Work out the finished part from the listing and answer in its coordinate system (mm). A direction names the side the tool comes from. Coordinates: 2 decimals unless noted, no trailing zeros. Loops run counter-clockwise (first coordinate to the right, second up) from the corner with the lowest first, then second, coordinate; pieces in that order, holes last. Notation, with made-up numbers: (26.25, -30) -> (50.25, -30) arc R14 cw to (50.25, -3) -> close; hole circle Ø6 at (45, -17.75). An arc over 180 degrees is marked (long way). Use a Markdown table: item, result.
from build123d import *

# Parameters (mm, degrees)
SKETCH1_R            = 5.5
SKETCH1_R_2          = 1.5
BOSS_EXTRUDE1_DEPTH  = 15
SKETCH3_W            = 9.999397818
SKETCH3_H            = 22.225224056
CUT_EXTRUDE1_DEPTH   = 5
FILLET1_R            = 1
FILLET1_OF_MIRROR1_R = 1
SKETCH4_R            = 7.5
BOSS_EXTRUDE2_DEPTH  = 3
SKETCH5_W            = 22
SKETCH5_H            = 7
CUT_EXTRUDE2_DEPTH   = 30.75172255
SKETCH6_R            = 4.5
CUT_EXTRUDE3_DEPTH   = 26.34097462
SKETCH7_R            = 4.5
CUT_EXTRUDE8_DEPTH   = 3
FILLET3_R            = 0.5
FILLET2_R            = 0.5


with BuildPart() as part:
    # Sketch1 → Boss-Extrude1 (new body)
    with BuildSketch(Plane.XY):
        with BuildLine():
            Line((-14.334802826, 9), (14.334802826, 9))
            ThreePointArc((14.334802826, 9), (17.163229951, 7.828427125), (18.334802826, 5))
            Line((18.334802826, 5), (18.334802826, -5))
            ThreePointArc((18.334802826, -5), (17.163229951, -7.828427125), (14.334802826, -9))
            Line((14.334802826, -9), (-14.334802826, -9))
            ThreePointArc((-14.334802826, -9), (-17.163229951, -7.828427125), (-18.334802826, -5))
            Line((-18.334802826, -5), (-18.334802826, 5))
            ThreePointArc((-18.334802826, 5), (-17.163229951, 7.828427125), (-14.334802826, 9))
        make_face()
        Circle(SKETCH1_R, mode=Mode.SUBTRACT)
        with Locations((-14.334802826, 0)):
            Circle(SKETCH1_R_2, mode=Mode.SUBTRACT)
        with Locations(Location((14.334802826, 0, 0), (0, 0, 180))):
            Circle(SKETCH1_R_2, mode=Mode.SUBTRACT)
    extrude(amount=BOSS_EXTRUDE1_DEPTH)

    # Sketch3 → Cut-Extrude1 (cut)
    with BuildSketch(Plane.XY.offset(15)):
        with Locations((-14.334501735, -0.429661625)):
            Rectangle(SKETCH3_W, SKETCH3_H)
    cut_extrude1 = extrude(amount=-CUT_EXTRUDE1_DEPTH, mode=Mode.SUBTRACT)

    # Fillet1
    fillet1_edges = [part.edges().sort_by_distance(p)[0] for p in [
        (-9.334802826, -9, 12.5),
        (-9.334802826, 0, 10),
        (-9.334802826, 9, 12.5),
        (-17.163229951, 7.828427125, 10),
        (-11.834802826, 9, 10),
        (-11.834802826, -9, 10),
        (-17.163229951, -7.828427125, 10),
        (-18.334802826, 0, 10),
        (-9.334802826, 0, 15),
    ]]
    fillet(fillet1_edges, radius=FILLET1_R)

    # Mirror1: Cut-Extrude1 across plane
    add(cut_extrude1.mirror(Plane(origin=(0, 0, 0), x_dir=(0, 0, 1), z_dir=(1, 0, 0))), mode=Mode.SUBTRACT)

    # Fillet1 of Mirror1
    fillet1_of_mirror1_edges = [part.edges().sort_by_distance(p)[0] for p in [
        (9.334802826, -9, 12.5),
        (9.334802826, 0, 10),
        (9.334802826, 9, 12.5),
        (17.163229951, 7.828427125, 10),
        (11.834802826, 9, 10),
        (11.834802826, -9, 10),
        (17.163229951, -7.828427125, 10),
        (18.334802826, 0, 10),
        (9.334802826, 0, 15),
    ]]
    fillet(fillet1_of_mirror1_edges, radius=FILLET1_OF_MIRROR1_R)

    # Sketch4 → Boss-Extrude2 (add)
    with BuildSketch(Plane.XY.offset(15)):
        Circle(SKETCH4_R)
    extrude(amount=-BOSS_EXTRUDE2_DEPTH)

    # Sketch5 → Cut-Extrude2 (cut, through all)
    with BuildSketch(Plane(origin=(0, 9, 0), x_dir=(1, 0, 0), z_dir=(0, 1, 0))):
        Rectangle(SKETCH5_W, SKETCH5_H)
    extrude(amount=-CUT_EXTRUDE2_DEPTH, mode=Mode.SUBTRACT)

    # Sketch6 → Cut-Extrude3 (cut, through all)
    with BuildSketch(Plane.XY.offset(15)):
        Circle(SKETCH6_R)
    extrude(amount=-CUT_EXTRUDE3_DEPTH, mode=Mode.SUBTRACT)

    # Sketch7 → Cut-Extrude8 (cut)
    with BuildSketch(Plane.XY.offset(10)):
        with Locations((-14.530374954, 0)):
            Circle(SKETCH7_R)
        with Locations((14.530374954, 0)):
            Circle(SKETCH7_R)
    extrude(amount=-CUT_EXTRUDE8_DEPTH, mode=Mode.SUBTRACT)

    # Fillet3
    fillet3_edges = [part.edges().sort_by_distance(p)[0] for p in [
        (11, -9, 1.75),
        (0, -9, 3.5),
        (11, 0, 3.5),
        (-11, -9, 1.75),
        (-11, 0, 3.5),
        (-11, 9, 1.75),
        (0, 9, 3.5),
        (11, 9, 1.75),
    ]]
    fillet(fillet3_edges, radius=FILLET3_R)

    # Fillet2
    fillet2_edges = [part.edges().sort_by_distance(p)[0] for p in [
        (-5.5, 0, 12),
    ]]
    fillet(fillet2_edges, radius=FILLET2_R)


solid = part.part
Q1. Section C-C on z = 8.5 is taken. Determine the outline of the cut face in (x, y), and give its area (3 significant figures).
Solved:
| item | result |
|---|---|
| outline | (-18.33, -5) arc R4 ccw to (-14.33, -9) -> (14.33, -9) arc R4 ccw to (18.33, -5) -> (18.33, -2.4) arc R4.5 cw (long way) to (18.33, 2.4) -> (18.33, 5) arc R4 ccw to (14.33, 9) -> (-14.33, 9) arc R4 ccw to (-18.33, 5) -> (-18.33, 2.4) arc R4.5 cw (long way) to (-18.33, -2.4) -> close; hole circle Ø11 at (0, 0) |
| area | 429 mm² |
Q2. Consider line 1 (X direction, y = 0, z = 8); line 2 (Z direction, x = -5, y = 3.5); line 3 (Z direction, x = -16, y = -5.5). Determine where each line is inside the solid, lowest interval first. Write a range as [from, to].
Solved:
| item | result |
|---|---|
| line 1 | [-10.03, -5.5], [5.5, 10.03] |
| line 2 | [3.5, 15] |
| line 3 | [0, 10] |
Q3. Section A-A on x = 0 is taken. Determine the outline of the cut face in (y, z), and give its area (3 significant figures).
Solved:
| item | result |
|---|---|
| outline | (-9, 4) arc R0.5 ccw to (-8.5, 3.5) -> (-5.5, 3.5) -> (-5.5, 11.5) arc R0.5 cw to (-5, 12) -> (-4.5, 12) -> (-4.5, 15) -> (-9, 15) -> close; (4.5, 12) -> (5, 12) arc R0.5 cw to (5.5, 11.5) -> (5.5, 3.5) -> (8.5, 3.5) arc R0.5 ccw to (9, 4) -> (9, 15) -> (4.5, 15) -> close |
| area | 86.5 mm² |
Q4. Section B-B on z = 4.75 is taken. Determine the outline of the cut face in (x, y).
Solved:
| item | result |
|---|---|
| outline | (-18.33, -5) arc R4 ccw to (-14.33, -9) -> (14.33, -9) arc R4 ccw to (18.33, -5) -> (18.33, 5) arc R4 ccw to (14.33, 9) -> (-14.33, 9) arc R4 ccw to (-18.33, 5) -> close; hole circle Ø3 at (-14.33, 0); hole circle Ø11 at (0, 0); hole circle Ø3 at (14.33, 0) |
Q5. Determine the mould class of faces 1 (the flat face through (16, 0, 0)), 2 (the cylindrical face through (10.033, 0.162, 8.521)), 3 (the cylindrical face through (-17.13, -7.86, 4.44)) for opening direction X: pulls with the +X half, pulls with the -X half, needs draft (parallel to the pull), parting line crosses it, or undercut.
Solved:
| item | result |
|---|---|
| face 1 | needs draft |
| face 2 | undercut |
| face 3 | pulls with the -X half |
Q6. Given pin 1 Ø4 at (x, y) = (-16, 1) entering from +Z; pin 2 Ø1.5 at (x, z) = (1, 3) entering from +Y; pin 3 Ø2.5 at (y, z) = (-1.5, 12.5) entering from +X, each flat-ended and moving along its own axis, determine where each tip first touches the part or whether it passes through.
Solved:
| item | result |
|---|---|
| pin 1 | z = 7 |
| pin 2 | y = 8.93 |
| pin 3 | x = 9.33 |
Q7. Section D-D on y = 0 is taken. State how many separate pieces and enclosed holes the cut face has, and give its area (3 significant figures).
Solved:
| item | result |
|---|---|
| separate pieces | 4 |
| enclosed holes | 0 |
| area | 171 mm² |
Q8. For faces 4 (the flat face through (11, 0, 2)), 5 (the cylindrical face through (9.05, -8.7, 13.03)), 6 (the cylindrical face through (-9.05, -8.7, 13.03)), 7 (the flat face through (-13, 6, 10)), determine the directions among +Z, -Z, +X, -X, +Y, -Y from which every point of the face is accessible in a straight line to the end or side of a thin tool.
Solved:
| item | result |
|---|---|
| face 4 | -Z, +Y, -Y |
| face 5 | +Z, +X, -Y |
| face 6 | +Z, -X, -Y |
| face 7 | +Z, -X, +Y, -Y |
